Geometry: final body of the model. Coordinates: model frame, mm. A direction names the side the tool comes from. Coordinates: 2 decimals unless noted, no trailing zeros. Write each loop counter-clockwise with the first axis right and the second up, starting at its lowest first coordinate (ties: lowest second). Pieces come first, ordered by that corner, then holes.
Autodesk Fusion 360 part; units mm, degrees
sketch "Sketch1" plane through (0, 0, 0) normal (0, 1, 0) x (1, 0, 0)
  circle A0 centre (0, 0) radius 37.5
  circle A1 centre (0, 0) radius 75
  line L0 (-75, 0) -> (-37.5, 0) construction
  circle A2 centre (-56.25, 0) radius 5
  line L1 (0, -75) -> (0, 75) construction
  circle A3 centre (56.25, 0) radius 5
  circle A4 centre (28.125, 48.7139) radius 5
  circle A5 centre (-28.125, 48.7139) radius 5
  circle A6 centre (-56.25, 0) radius 5
  circle A7 centre (-28.125, -48.7139) radius 5
  circle A8 centre (28.125, -48.7139) radius 5
  dimension "d1" = 75
  dimension "d2" = 150
  dimension "d3" = 10
  dimension "d5" = 360
extrude "Extrude1" add sketch "Sketch1" along normal blind 20
sketch "Sketch2" plane through (0, 0, 0) normal (0, 0, 1) x (1, 0, 0)
  line L0 (75, 20) -> (-75, 20)
  line L1 (-75, 0) -> (-75, 20)
  line L2 (75, 0) -> (-75, 0)
  line L3 (75, 0) -> (75, 20)
  line L4 (-50, 20) -> (50, 20)
  line L5 (-50, 20) -> (-50, 70)
  line L6 (50, 20) -> (50, 70)
  point P0 (0, 20)
  dimension "d8" = 100
  dimension "d9" = 50
sketch "Sketch3" plane through (0, 20, 0) normal (0, 1, 0) x (-1, 0, 0)
  circle A0 centre (28.125, 48.7139) radius 5
  circle A1 centre (-28.125, 48.7139) radius 5
  circle A2 centre (56.25, 0) radius 5
  circle A3 centre (0, 0) radius 37.5
  circle A4 centre (28.125, -48.7139) radius 5
  circle A5 centre (-56.25, 0) radius 5
  circle A6 centre (-28.125, -48.7139) radius 5
  circle A7 centre (0, 0) radius 75
  circle A8 centre (0, 0) radius 50
  dimension "d10" = 100
extrude "Extrude2" add sketch "Sketch3" along normal blind 50 contours A8
sketch "Sketch4" plane through (0, 70, 0) normal (0, 1, 0) x (-1, 0, 0)
  circle A0 centre (0, 0) radius 37.5
  circle A1 centre (0, 0) radius 50
sketch "Sketch5" plane through (0, 0, 0) normal (1, 0, 0) x (0, 1, 0)
  line L0 (70, -50) -> (70, 50)
  line L1 (20, 50) -> (70, 50)
  line L2 (20, 50) -> (20, 75)
  line L3 (0, 75) -> (20, 75)
  line L4 (0, 0) -> (0, 75)
  line L5 (0, -75) -> (0, 0)
  line L6 (0, -75) -> (20, -75)
  line L7 (20, -75) -> (20, -50)
  line L8 (20, -50) -> (70, -50)
  arc A0 (270, -200) -> (70, 0) centre (70, -200) ccw construction
  line L9 (20, 0) -> (70, 0)
  dimension "d13" = 200
sweep "Sweep1" add profiles "Sketch4" path "Sketch5" along A0 section 1
sketch "Sketch6" plane through (0, 0, -200) normal (0, 0, -1) x (1, 0, 0)
  circle A0 centre (0, -270) radius 37.5
  circle A1 centre (0, -270) radius 50
sketch "Sketch7" plane through (0, 0, 0) normal (0, 1, 0) x (1, 0, 0)
extrude "Extrude3" add sketch "Sketch6" along normal blind 50
sketch "Sketch8" plane through (0, 0, -250) normal (0, 0, -1) x (1, 0, 0)
  circle A0 centre (0, -270) radius 37.5
  circle A1 centre (0, -270) radius 50
  circle A2 centre (0, -270) radius 75
  line L0 (0, -270) -> (75, -270) construction
  circle A3 centre (56.25, -270) radius 5
  line L1 (0, -345) -> (0, -195) construction
  circle A4 centre (28.125, -221.2861) radius 5
  circle A5 centre (-28.125, -221.2861) radius 5
  circle A6 centre (-56.25, -270) radius 5
  circle A7 centre (-28.125, -318.7139) radius 5
  circle A8 centre (28.125, -318.7139) radius 5
  dimension "d23" = 150
  dimension "d24" = 10
  dimension "d25" = 56.25
  dimension "d27" = 360
extrude "Extrude4" add sketch "Sketch8" along normal blind 20 contours A1 | A2
Item 1: Section D-D, the plane y = 44. Output: boundary loops of the cut face in (x, z).
Derived:
outline: circle Ø100 at (0, 0); hole circle Ø75 at (0, 0)
Item 2: Material intervals for probe 1 along X at (y, z) = (15, 0); probe 2 along Y at (x, z) = (0, -214); probe 3 along Z at (x, y) = (0, 27), sorted ascending.
Derived:
probe 1: x = -75 to -61.25, -51.25 to -37.5, 37.5 to 51.25, 61.25 to 75
probe 2: y = 220 to 232.5, 307.5 to 320
probe 3: z = -50 to -37.5, 37.5 to 50
Item 3: Set-up query: faces 1 (the cylindrical face through (-2.47, 34.51, -37.42)), 2 (the cylindrical face through (-8.13, 233.39, -234.51)), 3 (the cylindrical face through (-47.69, 44.65, -15.02)), 4 (the cylindrical face through (-56.901, 274.957, -259.86)). Return all of +Z, -Z, +X, -X, +Y, -Y with unobstructed straight access to the full face (end or side cutting, diameter ignored); none if empty.
Derived:
face 1: -Y
face 2: -Z
face 3: none
face 4: +Z, -Z
Item 4: Section B-B, the plane x = -56.25. Output: boundary loops of the cut face in (y, z), plus the area to 3 significant figures.
Derived:
outline: (0, -49.61) - (20, -49.61) - (20, -5) - (0, -5) - close; (0, 5) - (20, 5) - (20, 49.61) - (0, 49.61) - close; (220.39, -270) - (265, -270) - (265, -250) - (220.39, -250) - close; (275, -270) - (319.61, -270) - (319.61, -250) - (275, -250) - close
area: 3,570 mm2
Item 5: Pull-direction query (X, two-part tool) for faces 5 (the cylindrical face through (-6.509, 319.575, -224.65)), 6 (the cylindrical face through (55.599, 274.957, -259.86)), 7 (the flat face through (16, 319, -250)); classes: released by +X, released by -X, zero draft, split by the parting line, or undercut.
Derived:
face 5: split by the parting line
face 6: undercut
face 7: zero draft
Item 6: Pin query (flat end, axial travel): pin 1 (16 mm diameter, centred on x = 28.12, y = 318.71, fed in from -Z); pin 2 (6 mm diameter, centred on x = -56.25, y = 270, fed in from +Z); pin 3 (12 mm diameter, centred on x = 0, z = -73.5, fed in from +Y); pin 4 (6 mm diameter, centred on x = 28.12, z = -48.71, fed in from +Y). Return the tip coordinate at first contact, or that it passes through.
Derived:
pin 1: stops at z = -270
pin 2: passes through
pin 3: stops at y = 289.04
pin 4: stops at y = 261.46
Item 7: Section C-C, the plane y = 270. State how many separate pieces and enclosed holes the cut face has, plus the area to 3 significant figures.
Derived:
separate pieces: 3
enclosed holes: 0
area: 7,000 mm2
